Can you work these out from the model? Positions are in its coordinate system, mm. Face numbers are marked on the shaded views. A direction names the side the tool comes from. Coordinates: 2 decimals unless noted, no trailing zeros. Loops run counter-clockwise (first coordinate to the right, second up) from the corner with the lowest first, then second, coordinate; pieces in that order, holes last.
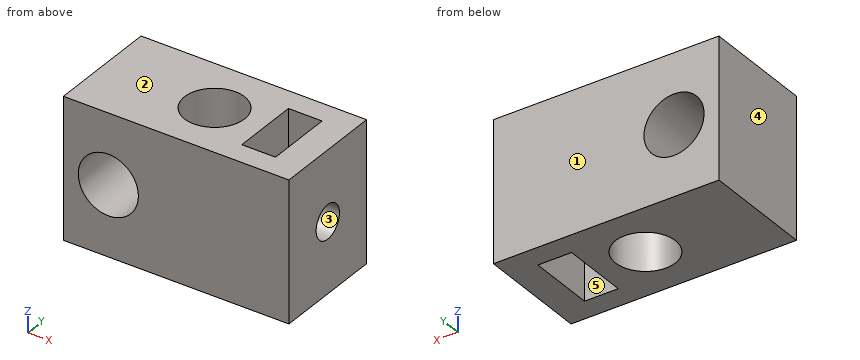
Autodesk Inventor part; units mm, degrees
ref_plane "YZ Plane" through (0, 0, 0) normal (1, 0, 0) x (0, 1, 0)
ref_plane "XZ Plane" through (0, 0, 0) normal (0, 1, 0) x (-1, 0, 0)
ref_plane "XY Plane" through (0, 0, 0) normal (0, 0, 1) x (1, 0, 0)
sketch "Sketch1" plane through (0, 0, 0) normal (0, 0, 1) x (1, 0, 0)
  circle A0 centre (0, 0) radius 2.675
  line L0 (-10, 5) -> (10.0805, 5)
  line L1 (10.0805, 5) -> (10.0805, -5)
  line L2 (10.0805, -5) -> (-10, -5)
  line L3 (-10, -5) -> (-10, 5)
  line L4 (7.5, -3) -> (4.5, -3)
  line L5 (4.5, -3) -> (4.5, 3)
  line L6 (4.5, 3) -> (7.5, 3)
  line L7 (7.5, 3) -> (7.5, -3)
  line L8 (7.5, -3) -> (4.5, 3) construction
  line L9 (4.5, -3) -> (7.5, 3) construction
  point P0 (6, 0)
  dimension "d0" = 5.35
  dimension "d1" = 5
  dimension "d2" = 5
  dimension "d3" = 10
  dimension "d4" = 3
  dimension "d5" = 6
  dimension "d6" = 6
extrude "Extrusion1" add sketch "Sketch1" along normal blind 12.5
sketch "Sketch2" plane through (10.0805, -5, 0) normal (1, 0, 0) x (0, 0, -1)
  point P0 (0, 5)
sketch "Sketch3" plane through (10.0805, -5, 0) normal (1, 0, 0) x (0, 0, -1)
  line L0 (-12.5, 2.325) -> (0, 2.325)
  line L1 (-12.5, 2.325) -> (0, 7.675)
  line L2 (-12.5, 7.675) -> (0, 7.675)
  circle A0 centre (-6.25, 5) radius 1.5
  point P0 (0, 5)
  dimension "d9" = 3
extrude "Extrusion2" cut sketch "Sketch3" against normal blind 10.25
sketch "Sketch4" plane through (-10, 5, 0) normal (0, 1, 0) x (1, 0, 0)
  circle A0 centre (4, -6.25) radius 2.675
  line L0 (0, 0) -> (0, -12.5)
  point P0 (10, 0)
  dimension "d12" = 5.35
  dimension "d13" = 4
extrude "Extrusion3" cut sketch "Sketch4" against normal blind 14
properties part number "CentralStabalizerShaft"
(1) If we mould it in two halves opening along Y, with no side actions, what happens to the marked faces 1, 2 and 3? For each: released by +Y, released by -Y, zero draft, split by the parting line, or undercut.
Check values:
face 1: released by +Y
face 2: zero draft
face 3: undercut
(2) I want a section at A-A on x = 7. Write out the boundary of the cut face in (y, z).
Check values:
outline: (-5, 0) - (-3, 0) - (-3, 12.5) - (-5, 12.5) - close; (3, 0) - (5, 0) - (5, 12.5) - (3, 12.5) - close
(3) Which directions (+Z, -Z, +X, -X, +Y, -Y) give clear straight access to the entire face, cutting with the end or side of a thin tool? Please do the marked faces 4 and 5.
Check values:
face 4: +Z, -Z, -X, +Y, -Y
face 5: +Z, -Z
(4) If I drill on probe 1 along Y at (x, z) = (8.35, 6.25); probe 2 along X at (y, z) = (2, 7.5); probe 3 along X at (y, z) = (-1.75, 11.75), over which ranges is the centre line in solid material (lowest first)?
Check values:
probe 1: y = -5 to -1.5, 1.5 to 5
probe 2: x = -10 to -8.36, -3.64 to -1.78, 1.78 to 4.5, 7.5 to 10.08
probe 3: x = -10 to -2.02, 2.02 to 4.5, 7.5 to 10.08
(5) I'm going to push a flat-ended pin straight in: pin 1 (5 mm diameter, centred on y = 0, z = 6.25, fed in from +X). Where does the tip first touch, or does it pass through?
Check values:
pin 1: stops at x = 10.08
(6) I want a section at C-C on y = -2. State how many separate pieces and enclosed holes the cut face has, then the cut area to 3 significant figures.
Check values:
separate pieces: 3
enclosed holes: 1
area: 147 mm2
